Model file for the job. Use its own axes, mm. A direction names the side the tool comes from. Round coordinates to 2 decimals unless told otherwise and drop trailing zeros. Loops run counter-clockwise (first coordinate to the right, second up) from the corner with the lowest first, then second, coordinate; pieces in that order, holes last. Notation, with made-up numbers: M -10,65 L 45,65 A29 ccw 45,85 Z; hole C 29,44.25 d6. An arc over 180 degrees is marked long. Use a Markdown table: item, result. Add a question column.
Q1. Tool access for faces 1 (the face through (0, 6.35, 7)), 2 (the face through (-7.638, 1.728, -0.774)), 3 (the face through (-5.49, 3.22, -5.86)), 4 (the face through (1.073, 4.622, -7.718)): list every direction of +Z, -Z, +X, -X, +Y, -Y with a clear straight run to the whole face (end or side of a thin tool).
Q2. Pin check, flat tips, straight feed: pin 1 (3.5 mm diameter, centred on x = 0, z = 11, fed in from +Y); pin 2 (4 mm diameter, centred on x = -4, z = -1.5, fed in from -Y); pin 3 (5 mm diameter, centred on x = -11.13, z = 0, fed in from -Y); pin 4 (2 mm diameter, centred on x = 1.5, y = 2, fed in from -Z). Stop position of each tip, or through.
Q3. Cut at C-C (x = 4). Give the cut face in (y, z).
Q4. Probe line 1 (X direction, y = 2.5, z = 0) (3 decimals); line 2 (Z direction, x = -10, y = 5.75); line 3 (X direction, y = 3.5, z = -6.5). List the from-to ranges inside material, lowest first. Write a range as from..to.
Q5. Cut at A-A (x = 0). Give the cut face in (y, z) (3 decimals), plus the area to 3 significant figures.
Q6. Mould opens along X. For faces 5 (the face through (-15.497, 3.131, -3.441)), 6 (the face through (10.26, 3.22, -6.13)), 7 (the face through (-7, 0, 0)) say: +X half, -X half, draft (parallel to the pull), parting line (faces both ways), or undercut.
Q7. Cut at B-B (z = 0). Give the cut face in (x, y) (3 decimals).
Q8. Cut at D-D (y = 4). State how many separate pieces and enclosed holes the cut face has, plus the area to 3 significant figures.
from build123d import *

# Parameters (mm, degrees)
SKETCH1_R                                      = 15.875
BOSS_EXTRUDE1_DEPTH                            = 6.35
SKETCH2_R                                      = 6.35
CUT_EXTRUDE1_DEPTH                             = 24.3313898
SKETCH11_R                                     = 2.286
CUT_EXTRUDE2_DEPTH                             = 24.3313898
CIRPATTERN3_COUNT                              = 2
CUT_EXTRUDE3_DEPTH                             = 24.3313898
CBORE_FOR_6_SOCKET_HEAD_CAP_SCREW2_D           = 3.6576
CBORE_FOR_6_SOCKET_HEAD_CAP_SCREW2_CBORE_D     = 7.14502
CBORE_FOR_6_SOCKET_HEAD_CAP_SCREW2_CBORE_DEPTH = 3.5052
CBORE_FOR_6_SOCKET_HEAD_CAP_SCREW1_D           = 3.6576
CBORE_FOR_6_SOCKET_HEAD_CAP_SCREW1_CBORE_D     = 7.14502
CBORE_FOR_6_SOCKET_HEAD_CAP_SCREW1_CBORE_DEPTH = 3.5052
CIRPATTERN5_COUNT                              = 2
CIRPATTERN6_COUNT                              = 2


with BuildPart() as part:
    # Sketch1 → Boss-Extrude1 (new body)
    with BuildSketch(Plane(origin=(0, 0, 0), x_dir=(1, 0, 0), z_dir=(0, 1, 0))):
        with Locations(Location((0, 0, 0), (0, 0, 270))):
            Circle(SKETCH1_R)
    extrude(amount=BOSS_EXTRUDE1_DEPTH)

    # Sketch2 → Cut-Extrude1 (cut, through all)
    with BuildSketch(Plane(origin=(0, 6.35, 0), x_dir=(1, 0, 0), z_dir=(0, 1, 0))):
        with Locations(Location((0, 0, 0), (0, 0, 270))):
            Circle(SKETCH2_R)
    extrude(amount=-CUT_EXTRUDE1_DEPTH, mode=Mode.SUBTRACT)

    # Sketch11 → Cut-Extrude2 (cut, through all)
    with BuildSketch(Plane(origin=(0, 6.35, 0), x_dir=(1, 0, 0), z_dir=(0, 1, 0))):
        with Locations(Location((8.328911597, 7.35641814, 0), (0, 0, 270))):
            Circle(SKETCH11_R)
    cut_extrude2 = extrude(amount=-CUT_EXTRUDE2_DEPTH, mode=Mode.SUBTRACT)

    # CirPattern3: Cut-Extrude2 ×2 about axis
    cirpattern3_axis = Axis((0, 0, 0), (0, 1, 0))
    for i in range(1, CIRPATTERN3_COUNT):
        add(cut_extrude2.rotate(cirpattern3_axis, i * 360 / CIRPATTERN3_COUNT), mode=Mode.SUBTRACT)

    # Sketch12 → Cut-Extrude3 (cut, through all)
    with BuildSketch(Plane(origin=(0, 6.35, 0), x_dir=(1, 0, 0), z_dir=(0, 1, 0))):
        with BuildLine():
            Line((-6.39758264, 4.883452605), (-4.554151289, 6.87011727))
            ThreePointArc((-4.554151289, 6.87011727), (-4.0916663, 6.887412726), (-4.074370844, 6.424927737))
            Line((-4.074370844, 6.424927737), (-5.917802195, 4.438263073))
            ThreePointArc((-5.917802195, 4.438263073), (-6.380287183, 4.420967617), (-6.39758264, 4.883452605))
        make_face()
    extrude(amount=-CUT_EXTRUDE3_DEPTH, mode=Mode.SUBTRACT)

    # CBORE for #6 Socket Head Cap Screw2 (through all)
    with Locations(Plane(origin=(11.1252, 0, 0), x_dir=(0, 0, -1), z_dir=(0, -1, 0))):
        with Locations((0, 0)):
            cbore_for_6_socket_head_cap_screw2 = CounterBoreHole(CBORE_FOR_6_SOCKET_HEAD_CAP_SCREW2_D / 2, CBORE_FOR_6_SOCKET_HEAD_CAP_SCREW2_CBORE_D / 2, CBORE_FOR_6_SOCKET_HEAD_CAP_SCREW2_CBORE_DEPTH)

    # CBORE for #6 Socket Head Cap Screw1 (through all)
    with Locations(Plane(origin=(0, 6.35, -11.1252), x_dir=(0, 0, 1), z_dir=(0, 1, 0))):
        with Locations((0, 0)):
            cbore_for_6_socket_head_cap_screw1 = CounterBoreHole(CBORE_FOR_6_SOCKET_HEAD_CAP_SCREW1_D / 2, CBORE_FOR_6_SOCKET_HEAD_CAP_SCREW1_CBORE_D / 2, CBORE_FOR_6_SOCKET_HEAD_CAP_SCREW1_CBORE_DEPTH)

    # CirPattern5: CBORE for #6 Socket Head Cap Screw1 ×2 about axis
    cirpattern5_axis = Axis((0, 0, 0), (0, 1, 0))
    for i in range(1, CIRPATTERN5_COUNT):
        add(cbore_for_6_socket_head_cap_screw1.rotate(cirpattern5_axis, i * 360 / CIRPATTERN5_COUNT), mode=Mode.SUBTRACT)

    # CirPattern6: CBORE for #6 Socket Head Cap Screw2 ×2 about axis
    cirpattern6_axis = Axis((0, 0, 0), (0, 1, 0))
    for i in range(1, CIRPATTERN6_COUNT):
        add(cbore_for_6_socket_head_cap_screw2.rotate(cirpattern6_axis, i * 360 / CIRPATTERN6_COUNT), mode=Mode.SUBTRACT)


solid = part.part
Checked values:
| question | item | result |
|---|---|---|
| 1 | face 1 | +Z, -Z, +X, -X, +Y |
| 1 | face 2 | -Y |
| 1 | face 3 | +Y, -Y |
| 1 | face 4 | +Y |
| 2 | pin 1 | stops at y = 2.84 |
| 2 | pin 2 | passes through |
| 2 | pin 3 | stops at y = 3.51 |
| 2 | pin 4 | stops at z = -15.87 |
| 3 | outline | M 0,-15.36 L 6.35,-15.36 L 6.35,-4.93 L 0,-4.93 Z; M 0,4.93 L 6.35,4.93 L 6.35,15.36 L 0,15.36 Z |
| 4 | line 1 | x = -15.875..-14.698, -7.553..-6.35, 6.35..7.553, 14.698..15.875 |
| 4 | line 2 | z = -12.33..-1.44, 1.44..5.8, 8.92..12.33 |
| 4 | line 3 | x = -14.48..-4.9, -4.02..6.21, 10.45..14.48 |
| 5 | outline | M 0,-15.875 L 6.35,-15.875 L 6.35,-14.698 L 2.845,-14.698 L 2.845,-12.954 L 0,-12.954 Z; M 0,-9.296 L 2.845,-9.296 L 2.845,-7.553 L 6.35,-7.553 L 6.35,-6.35 L 0,-6.35 Z; M 0,6.35 L 6.35,6.35 L 6.35,7.553 L 2.845,7.553 L 2.845,9.296 L 0,9.296 Z; M 0,12.954 L 2.845,12.954 L 2.845,14.698 L 6.35,14.698 L 6.35,15.875 L 0,15.875 Z |
| 5 | area | 50.1 mm^2 |
| 6 | face 5 | parting line |
| 6 | face 6 | undercut |
| 6 | face 7 | draft |
| 7 | outline | M -15.875,0 L -14.698,0 L -14.698,3.505 L -12.954,3.505 L -12.954,6.35 L -15.875,6.35 Z; M -9.296,3.505 L -7.553,3.505 L -7.553,0 L -6.35,0 L -6.35,6.35 L -9.296,6.35 Z; M 6.35,0 L 7.553,0 L 7.553,3.505 L 9.296,3.505 L 9.296,6.35 L 6.35,6.35 Z; M 12.954,3.505 L 14.698,3.505 L 14.698,0 L 15.875,0 L 15.875,6.35 L 12.954,6.35 Z |
| 8 | separate pieces | 1 |
| 8 | enclosed holes | 8 |
| 8 | area | 529 mm^2 |
